Check sheet for the modelled part. Datum: model origin and axes. Units: mm. Give positions to 0.01 mm unless a question says otherwise; leave off trailing zeros. Order: outer loops, then holes, each group sorted by start corner. A loop starts at its lowest first (then second) coordinate and runs counter-clockwise, first axis right, second up.
Item 1: Gauge pin test, flat end, axial feed: P1, Ø8, axis at x = -5.5, z = 12.5, coming from the -Y side. Record the tip position at first contact, or that the pin passes through.
Item 2: Sectioned sample at B-B on y = 0.4. Count the separate pieces of the cut face and the enclosed holes in it, and give its area (3 significant figures).
Item 3: Material ranges on line 1 along X through (y, z) = (0.7, 0); line 2 along X through (y, z) = (0.65, -27.5); line 3 along X through (y, z) = (0.75, 25.5), recorded low to high.
Item 4: Sectioned sample at D-D on z = -30. Record the boundary of the cut face in (x, y), and give its area (3 significant figures).
Item 5: Sectioned sample at A-A on z = 0. Record the boundary of the cut face in (x, y).
Item 6: Sectioned sample at C-C on x = -31. Record the boundary of the cut face in (y, z), and give its area (3 significant figures).
from build123d import *

# Parameters (mm, degrees)
SKETCH1_R           = 1.5
SKETCH1_R_2         = 3
BOSS_EXTRUDE1_DEPTH = 2


with BuildPart() as part:
    # Sketch1 → Boss-Extrude1 (new body)
    with BuildSketch(Plane(origin=(0, 0, 0), x_dir=(1, 0, 0), z_dir=(0, 1, 0))):
        with BuildLine():
            ThreePointArc((27.5, -7.5), (35, 0), (27.5, 7.5))
            add(Edge.make_bspline(
                [(27.5, 7.5), (5.834523779, 5.834523779), (7.5, 27.5)],
                knots=[0, 0, 0, 1, 1, 1], degree=2))
            ThreePointArc((7.5, 27.5), (0, 35), (-7.5, 27.5))
            add(Edge.make_bspline(
                [(-7.5, 27.5), (-5.834523779, 5.834523779), (-27.5, 7.5)],
                knots=[0, 0, 0, 1, 1, 1], degree=2))
            ThreePointArc((-27.5, 7.5), (-35, 0), (-27.5, -7.5))
            add(Edge.make_bspline(
                [(-27.5, -7.5), (-5.834523779, -5.834523779), (-7.5, -27.5)],
                knots=[0, 0, 0, 1, 1, 1], degree=2))
            ThreePointArc((-7.5, -27.5), (0, -35), (7.5, -27.5))
            add(Edge.make_bspline(
                [(7.5, -27.5), (5.834523779, -5.834523779), (27.5, -7.5)],
                knots=[0, 0, 0, 1, 1, 1], degree=2))
        make_face()
        with Locations(Location((0, 27.5, 0), (0, 0, 270))):
            Circle(SKETCH1_R, mode=Mode.SUBTRACT)
        with Locations(Location((-27.5, 0, 0), (0, 0, 270))):
            Circle(SKETCH1_R, mode=Mode.SUBTRACT)
        with Locations(Location((27.5, 0, 0), (0, 0, 270))):
            Circle(SKETCH1_R, mode=Mode.SUBTRACT)
        with Locations(Location((0, -27.5, 0), (0, 0, 270))):
            Circle(SKETCH1_R, mode=Mode.SUBTRACT)
        with Locations(Location((0, 0, 0), (0, 0, 270))):
            Circle(SKETCH1_R_2, mode=Mode.SUBTRACT)
    extrude(amount=BOSS_EXTRUDE1_DEPTH)


solid = part.part
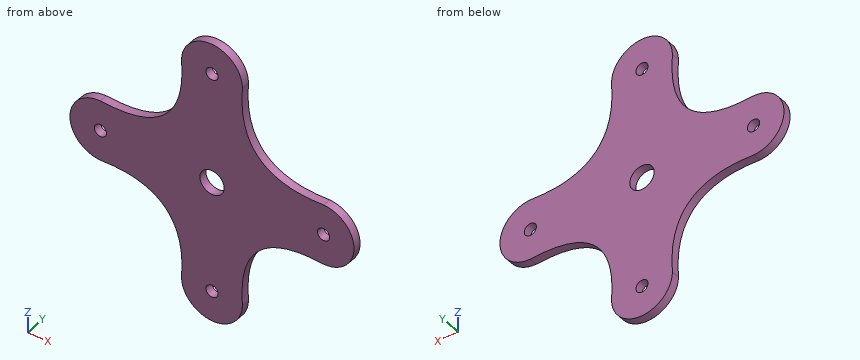
Report:
1. P1: stops at y = 0
2. separate pieces: 1
2. enclosed holes: 5
2. area: 1,900 mm2
3. line 1: x = -35 to -29, -26 to -3, 3 to 26, 29 to 35
3. line 2: x = -7.5 to -1.5, 1.5 to 7.5
3. line 3: x = -7.39 to 7.39
4. outline: (-7.07, 0) - (7.07, 0) - (7.07, 2) - (-7.07, 2) - close
4. area: 28.3 mm2
5. outline: (-35, 0) - (-29, 0) - (-29, 2) - (-35, 2) - close; (-26, 0) - (-3, 0) - (-3, 2) - (-26, 2) - close; (3, 0) - (26, 0) - (26, 2) - (3, 2) - close; (29, 0) - (35, 0) - (35, 2) - (29, 2) - close
6. outline: (0, -6.63) - (2, -6.63) - (2, 6.63) - (0, 6.63) - close
6. area: 26.5 mm2
